Part print with two shaded views. Sizes in mm from the minimum x, y, z corner. A direction names the side the tool comes from. Round coordinates to 2 decimals unless told otherwise and drop trailing zeros. Write each loop counter-clockwise with the first axis right and the second up, starting at its lowest first coordinate (ties: lowest second). Pieces come first, ordered by that corner, then holes. Notation, with made-up numbers: M 41,-38.75 L 48,-38.75 A34 cw 48,-5.75 Z; hole C 71.25,40.25 d8. An arc over 180 degrees is marked long. Use one line per item in the form item = value. Start each with the question number.
Item 1: Mould opens along Z. For the marked faces 3, 4, 5 and 6 say: +Z half, -Z half, draft (parallel to the pull), parting line (faces both ways), or undercut.
Item 2: Cut at C-C, the plane y = 263. Give the cut face in (x, z), then the cut area to 3 significant figures.
Item 3: Which spindle directions (+Z, -Z, +X, -X, +Y, -Y) get a long thin tool onto all of the face, cutting with end or side? Do the marked faces 1 and 2. Say none if no direction does.
Item 4: Cut at B-B, the plane x = 1913. Give the cut face in (y, z).
Item 5: Cut at A-A, the plane z = 279.5. Give the cut face in (x, y), then the cut area to 3 significant figures.
Item 6: Probe L1, parallel to X at y = 261, z = 255; L2, parallel to Z at x = 885, y = 258.5. List the from-to ranges inside material, lowest first.
Item 7: Flat gauge pin, fed straight in: pin 1 Ø1.5 at (x, y) = (2082, 322) entering from -Z. Where does the tip first touch, or does it go through?
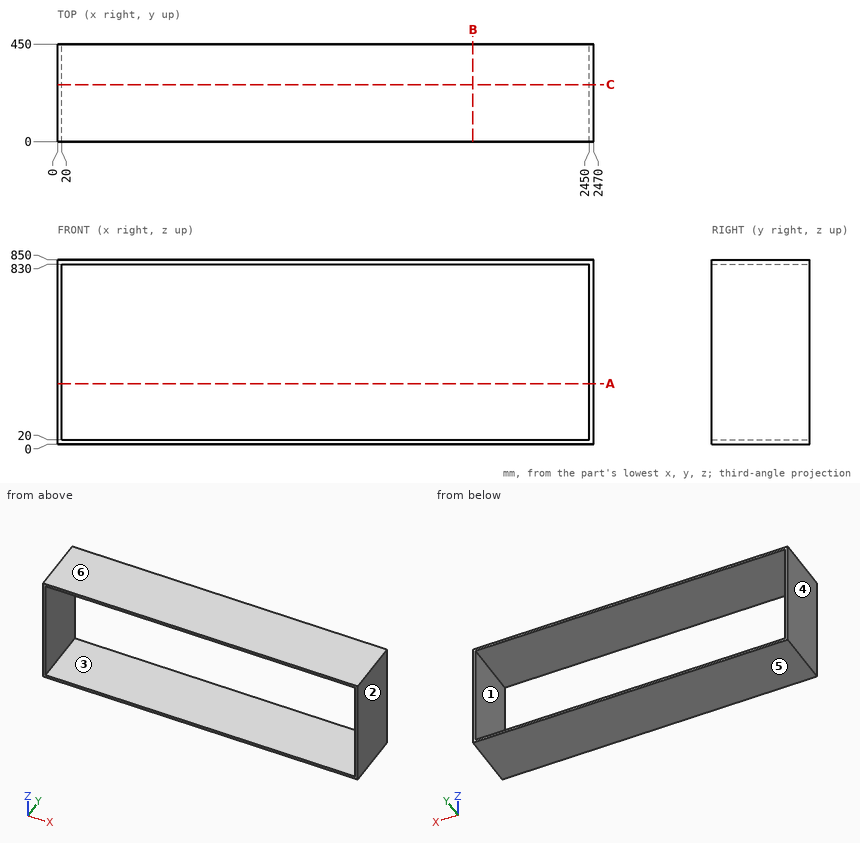
Model answer:
q1.face_3 = undercut
q1.face_4 = draft
q1.face_5 = -Z half
q1.face_6 = +Z half
q2.outline = M 0,0 L 2470,0 L 2470,850 L 0,850 Z; hole M 20,20 L 2450,20 L 2450,830 L 20,830 Z
q2.area = 131,000 mm²
q3.face_1 = +Y, -Y
q3.face_2 = +Z, -Z, +X, +Y, -Y
q4.outline = M 0,0 L 450,0 L 450,20 L 0,20 Z; M 0,830 L 450,830 L 450,850 L 0,850 Z
q5.outline = M 0,0 L 20,0 L 20,450 L 0,450 Z; M 2450,0 L 2470,0 L 2470,450 L 2450,450 Z
q5.area = 18,000 mm²
q6.L1 = 0 to 20, 2450 to 2470
q6.L2 = 0 to 20, 830 to 850
q7.pin_1 = 0
